Input: part model. Units: mm. Frame: model coordinates. A direction names the side the tool comes from. Give positions to 0.01 mm unless a question says otherwise; leave off trailing zeros. Loops run counter-clockwise (first coordinate to the right, second up) from the corner with the lowest first, then second, coordinate; pieces in that order, holes last. Notation, with made-up numbers: (45, 64) - (80, 64) arc R28 cw to (80, 102) - close; hole circle Ø3 at (-21, 42). An arc over 180 degrees is marked (long way). One line per item, written item: value.
from build123d import *

# Parameters (mm, degrees)
ESQUISSE1_R             = 4
BOSS_EXTRU_1_DEPTH      = 10.5
ESQUISSE2_W             = 8.8
ESQUISSE2_H             = 10.8
BOSS_EXTRU_2_DEPTH      = 3.3
ESQUISSE3_W             = 10.5
ESQUISSE3_H             = 5.9
BOSS_EXTRU_3_DEPTH      = 8.8
ESQUISSE4_R             = 3
ENL_V_MAT_EXTRU_1_DEPTH = 12
ESQUISSE5_R             = 0.3
BOSS_EXTRU_4_DEPTH      = 11.8


# Read off the part's stored shape, not the designer's step: Dôme1
with BuildPart() as part:
    # Esquisse1 → Boss.-Extru.1 (new body)
    with BuildSketch(Plane.XY):
        with Locations(Location((0, 0, 0), (0, 0, 180))):
            Circle(ESQUISSE1_R)
    extrude(amount=BOSS_EXTRU_1_DEPTH)

    # Esquisse2 → Boss.-Extru.2 (add)
    with BuildSketch(Plane.XY.offset(10.5)):
        with Locations((0, -0.6)):
            Rectangle(ESQUISSE2_W, ESQUISSE2_H)
    extrude(amount=BOSS_EXTRU_2_DEPTH)

    # Esquisse3 → Boss.-Extru.3 (add)
    with BuildSketch(Plane(origin=(4.4, 0, 0), x_dir=(0, 0, -1), z_dir=(1, 0, 0))):
        with Locations((-5.25, -2.95)):
            Rectangle(ESQUISSE3_W, ESQUISSE3_H)
    extrude(amount=-BOSS_EXTRU_3_DEPTH)

    # Esquisse4 → Enlèv. mat.-Extru.1 (cut)
    with BuildSketch(Plane.XY.offset(13.8)):
        Circle(ESQUISSE4_R)
    extrude(amount=-ENL_V_MAT_EXTRU_1_DEPTH, mode=Mode.SUBTRACT)

    # Esquisse5 → Boss.-Extru.4 (add)
    with BuildSketch(Plane.XY.offset(1.8)):
        Circle(ESQUISSE5_R)
    extrude(amount=BOSS_EXTRU_4_DEPTH)

    # Dôme1 outline → Dôme1 (revolve)
    with BuildSketch(Plane.XZ):
        with BuildLine():
            Line((0, 13.6), (0.3, 13.6))
            ThreePointArc((0.3, 13.6), (0.158113883, 13.674341649), (0, 13.7))
            Line((0, 13.7), (0, 13.6))
        make_face()
    revolve(axis=Axis((0, 0, 0), (0, 0, 1)))


solid = part.part
Item 1: Section A-A, the plane z = 10.25. Output: boundary loops of the cut face in (x, y).
Verdict:
outline: (-4.4, -5.9) - (4.4, -5.9) - (4.4, 0) - (4, 0) arc R4 ccw to (-4, 0) - (-4.4, 0) - close; circle Ø0.6 at (0, 0); hole circle Ø6 at (0, 0)
Item 2: Draft query along Y for faces 1 (the face through (-3, 0, 8)), 2 (the face through (-4.4, -2, 9)), 3 (the face through (0, -5.9, 5)), 4 (the face through (0, 4, 5)). Return one class per face: pulls with the +Y half, pulls with the -Y half, needs draft (parallel to the pull), parting line crosses it, or undercut.
Verdict:
face 1: undercut
face 2: needs draft
face 3: pulls with the -Y half
face 4: pulls with the +Y half
Item 3: Material intervals for L1, parallel to Y at x = 0, z = 8; L2, parallel to Z at x = -1.5, y = 2.5; L3, parallel to X at y = 1, z = 12, sorted ascending.
Verdict:
L1: y = -5.9 to -3, -0.3 to 0.3, 3 to 4
L2: z = 0 to 1.8
L3: x = -4.4 to -2.83, 2.83 to 4.4
Item 4: Section C-C, the plane x = 0. Output: boundary loops of the cut face in (y, z), and give its area (3 significant figures).
Verdict:
outline: (-6, 10.5) - (-5.9, 10.5) - (-5.9, 0) - (4, 0) - (4, 10.5) - (4.8, 10.5) - (4.8, 13.8) - (3, 13.8) - (3, 1.8) - (0.3, 1.8) - (0.3, 13.6) arc R0.5 ccw to (-0.3, 13.6) - (-0.3, 1.8) - (-3, 1.8) - (-3, 13.8) - (-6, 13.8) - close
area: 74.7 mm^2
Item 5: Access query for faces 5 (the face through (1, 0, 1.8)), 6 (the face through (-1.04, 4.03, 10.5)), 7 (the face through (-1, -3, 13.8)). Directions: +Z, -Z, +X, -X, +Y, -Y. A direction counts if a zero-diameter tool reaches every point of the face in a straight line with its end or side. Return the directions, or none.
Verdict:
face 5: +Z
face 6: -Z, +Y
face 7: +Z, +X, -X, +Y, -Y
Item 6: Pin query (flat end, axial travel): P1, Ø1, axis at x = -2, z = 3, coming from the -Y side; P2, Ø4, axis at x = -2.5, z = 6, coming from the +Y side. Return the tip coordinate at first contact, or that it passes through.
Verdict:
P1: stops at y = -5.9
P2: stops at y = 3.97
Item 7: Section B-B, the plane y = -2.75. Output: boundary loops of the cut face in (x, z).
Verdict:
outline: (-4.4, 0) - (4.4, 0) - (4.4, 13.8) - (1.2, 13.8) - (1.2, 1.8) - (-1.2, 1.8) - (-1.2, 13.8) - (-4.4, 13.8) - close
Item 8: Section D-D, the plane y = 3.5. Output: boundary loops of the cut face in (x, z), and give its area (3 significant figures).
Verdict:
outline: (-4.4, 10.5) - (-1.94, 10.5) - (-1.94, 0) - (1.94, 0) - (1.94, 10.5) - (4.4, 10.5) - (4.4, 13.8) - (-4.4, 13.8) - close
area: 69.7 mm^2
